from build123d import *

# Parameters (mm, degrees)
F0_W     = 85
F0_H     = 23
F1_DEPTH = 3
F2_W     = 3
F2_H     = 23
F3_DEPTH = 24
F4_W     = 3
F4_H     = 23
F5_DEPTH = 25
F6_R     = 4
F6_R_2   = 2
F7_DEPTH = 100


with BuildPart() as f1:
    # F0 (on Top) → F1 (new body)
    with BuildSketch(Plane.XY):
        with Locations((42.5, 11.5)):
            Rectangle(F0_W, F0_H)
        with BuildLine():
            Line((85, 0), (0, 0))
            Line((0, 0), (0, -10))
            Line((0, -10), (0, -65))
            ThreePointArc((0, -65), (1.464466, -68.535534), (5, -70))
            Line((5, -70), (7.5, -70))
            ThreePointArc((7.5, -70), (11.035534, -68.535534), (12.5, -65))
            Line((12.5, -65), (12.5, -15))
            ThreePointArc((12.5, -15), (13.964466, -11.464466), (17.5, -10))
            Line((17.5, -10), (67.5, -10))
            ThreePointArc((67.5, -10), (71.035534, -11.464466), (72.5, -15))
            Line((72.5, -15), (72.5, -65))
            ThreePointArc((72.5, -65), (73.964466, -68.535534), (77.5, -70))
            Line((77.5, -70), (80, -70))
            ThreePointArc((80, -70), (83.535534, -68.535534), (85, -65))
            Line((85, -65), (85, -10))
            Line((85, -10), (85, 0))
        make_face()
    extrude(amount=F1_DEPTH)

    # F2 (on face) → F3 (join)
    with BuildSketch(Plane.XY.offset(3)):
        with Locations((1.5, 11.5)):
            Rectangle(F2_W, F2_H)
        with Locations((83.5, 11.5)):
            Rectangle(F2_W, F2_H)
    extrude(amount=F3_DEPTH)

    # F4 (on face) → F5 (join)
    with BuildSketch(Plane.XY.offset(27)):
        with Locations((1.5, 11.5)):
            Rectangle(F4_W, F4_H)
    extrude(amount=F5_DEPTH)

    # F6 (on face) → F7 (cut)
    with BuildSketch(Plane.YZ.offset(85)):
        with Locations((11.5, 13.5)):
            Circle(F6_R)
        with Locations((19.713903, 13.5)):
            Circle(F6_R_2)
        with Locations((17.308106, 19.308106)):
            Circle(F6_R_2)
        with Locations((11.5, 21.713903)):
            Circle(F6_R_2)
        with Locations((5.691894, 19.308106)):
            Circle(F6_R_2)
        with Locations((3.286097, 13.5)):
            Circle(F6_R_2)
        with Locations((5.691894, 7.691894)):
            Circle(F6_R_2)
        with Locations((11.5, 5.286097)):
            Circle(F6_R_2)
        with Locations((17.308106, 7.691894)):
            Circle(F6_R_2)
    extrude(amount=-F7_DEPTH, mode=Mode.SUBTRACT)


solid = f1.part
The listing builds one solid part. Answer for the finished solid, in the listing's coordinates (mm). A direction names the side the tool comes from. Coordinates: 2 decimals unless noted, no trailing zeros. Write each loop counter-clockwise with the first axis right and the second up, starting at its lowest first coordinate (ties: lowest second). Pieces come first, ordered by that corner, then holes. Notation, with made-up numbers: (-6.5, 57.25) - (25.5, 57.25) arc R22 cw to (25.5, 86.25) - close; hole circle Ø9 at (20.25, 53.25). An arc over 180 degrees is marked (long way). Answer as CSV lines item,"result".
1. Find section D-D (x = 54). Give the vertices of the cut face in (y, z).
Computed values:
outline,"(-10, 0) - (23, 0) - (23, 3) - (-10, 3) - close"
2. Given P1, Ø3, axis at y = 11.5, z = 5.29, coming from the +X side; P2, Ø2.5, axis at x = 1, z = 39.5, coming from the -Y side; P3, Ø12, axis at x = 70, y = -15.5, coming from the +Z side, each flat-ended and moving along its own axis, determine where each tip first touches the part or whether it passes through.
Computed values:
P1,"passes through"
P2,"stops at y = 0"
P3,"stops at z = 3"
3. Find section B-B (y = -56.5). Give the vertices of the cut face in (x, z), plus the area to 3 significant figures.
Computed values:
outline,"(0, 0) - (12.5, 0) - (12.5, 3) - (0, 3) - close; (72.5, 0) - (85, 0) - (85, 3) - (72.5, 3) - close"
area,"75.0 mm²"
4. Determine the mould class of faces 4 (the flat face through (12.5, -40, 1)), 5 (the flat face through (36, 23, 2.8)), 6 (the cylindrical face through (83.521, 20.789, 15.186)) for opening direction Y: +Y half, -Y half, draft (parallel to the pull), parting line (faces both ways), or undercut.
Computed values:
face 4,"draft"
face 5,"+Y half"
face 6,"undercut"
5. Find section A-A (z = 13.5). Give the number of separate pieces and of enclosed holes in the cut face, plus the area to 3 significant figures.
Computed values:
separate pieces,"8"
enclosed holes,"0"
area,"42.0 mm²"
6. A tool of negligible diameter and unlimited length cuts with its end or side. For faces 1 (the flat face through (83, 12, 27)), 2 (the flat face through (3, 11, 27)), 3 (the flat face through (85, 2, 10)), from which of +Z, -Z, +X, -X, +Y, -Y can it reach the whole face along a straight path? Write none if from no direction.
Computed values:
face 1,"+Z, +X, +Y, -Y"
face 2,"+Z, +Y, -Y"
face 3,"+Z, -Z, +X, +Y, -Y"
7. Straight lines are drawn through the part: line 1 (Z direction, x = 1.6, y = 11.5); line 2 (Y direction, x = 1, z = 13); line 3 (X direction, y = 1, z = 23). For each, find the intervals that lie inside material, in ascending order. Write a range as [from, to].
Computed values:
line 1,"z = [0, 3.29], [7.29, 9.5], [17.5, 19.71], [23.71, 52]"
line 2,"y = [0, 1.35], [5.22, 7.53], [15.47, 17.78], [21.65, 23]"
line 3,"x = [0, 3], [82, 85]"
